Read the model definition and answer for the solid it produces. Units are mm, in the model's axes. Face numbers are marked on the shaded views. A direction names the side the tool comes from. Give positions to 0.01 mm unless a question says otherwise; leave off trailing zeros. Order: outer loops, then holes, each group sorted by start corner. A loop starts at its lowest first (then second) coordinate and runs counter-clockwise, first axis right, second up. Notation, with made-up numbers: (2.25, -37) - (13.25, -37) arc R8 cw to (13.25, -30) - close; hole circle Ø7 at (7, -30). An arc over 180 degrees is marked (long way). Use a Markdown table: item, result. Add a question column.
1. A cutting plane is placed at C-C on x = 36. Determine the outline of the cut face in (y, z), and give its area (3 significant figures).
2. A cutting plane is placed at B-B on z = 13. State how many separate pieces and enclosed holes the cut face has, and give its area (3 significant figures).
3. Consider L1, parallel to X at y = 1.45, z = -4; L2, parallel to Z at x = 62, y = 1.3; L3, parallel to Y at x = 28, z = -6. Determine where each line is inside the solid, lowest interval first.
4. Flat-ended cylindrical pins translate along their axes: P1, Ø9.5, axis at x = 37.36, z = 2.61, coming from the -Y side; P2, Ø1, axis at x = 7.5, z = 11.5, coming from the -Y side. Find the tip coordinate at first contact, or state that the pin passes through.
5. A cutting plane is placed at D-D on x = 67.5. Determine the outline of the cut face in (y, z), and give its area (4 significant figures).
6. Which of the six approach directions +Z, -Z, +X, -X, +Y, -Y give full straight-line access (tool end or side, diameter ignored) to the marked faces 3 and 4?
7. A cutting plane is placed at A-A on x = 17. Determine the outline of the cut face in (y, z).
8. For a pull along Z with two mould halves and no side action, classify the marked faces 1 and 2 as released by +Z, released by -Z, zero draft, split by the parting line, or undercut.
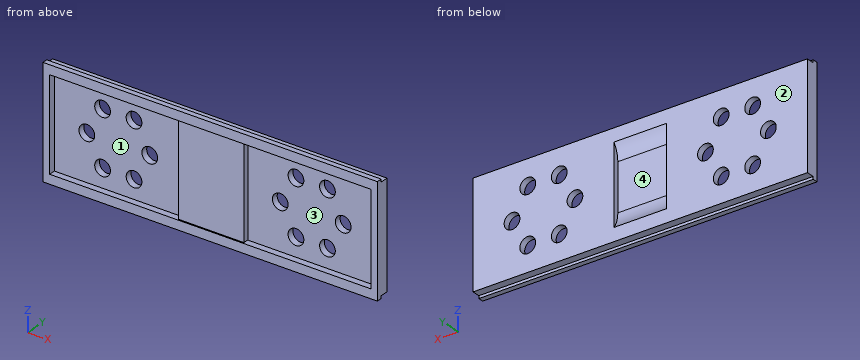
```python
from build123d import *

# Parameters (mm, degrees)
SKETCH1_W           = 127.5
SKETCH1_H           = 42
BOSS_EXTRUDE1_DEPTH = 5
SKETCH2_W           = 127.5
SKETCH2_H           = 1
CUT_EXTRUDE1_DEPTH  = 3
SKETCH7_W           = 20
SKETCH7_H           = 30
CUT_EXTRUDE5_DEPTH  = 2
SHELL8_START        = -14.893859366
SHELL8_DEPTH        = 35
FILLET3_R           = 10
FILLET4_R           = 10
SKETCH10_R          = 3
CUT_EXTRUDE6_DEPTH  = 2.5


# Read off the part's stored shape, not the designer's step: Shell8
with BuildPart() as part:
    # Sketch1 → Boss-Extrude1 (new body)
    with BuildSketch(Plane(origin=(0, 0, 0), x_dir=(1, 0, 0), z_dir=(0, 1, 0))):
        with Locations((12.48267617, -2.606140634)):
            Rectangle(SKETCH1_W, SKETCH1_H)
    extrude(amount=BOSS_EXTRUDE1_DEPTH)

    # Sketch2 → Cut-Extrude1 (cut)
    with BuildSketch(Plane(origin=(0, 5, 0), x_dir=(1, 0, 0), z_dir=(0, 1, 0))):
        with Locations((12.48267617, 17.893859366)):
            Rectangle(SKETCH2_W, SKETCH2_H)
        with Locations((12.48267617, -23.106140634)):
            Rectangle(SKETCH2_W, SKETCH2_H)
    extrude(amount=-CUT_EXTRUDE1_DEPTH, mode=Mode.SUBTRACT)

    # Sketch7 → Cut-Extrude5 (cut)
    with BuildSketch(Plane(origin=(0, 5, 0), x_dir=(1, 0, 0), z_dir=(0, 1, 0))):
        with Locations((12.48267617, -2.606140634)):
            Rectangle(SKETCH7_W, SKETCH7_H)
    extrude(amount=-CUT_EXTRUDE5_DEPTH, mode=Mode.SUBTRACT)

    # Shell8 outline → Shell8 (cut)
    with BuildSketch(Plane.XY.offset(SHELL8_START)):
        Polygon((-0.01732383, 0.5), (-0.01732383, 2.5), (-48.76732383, 2.5), (-48.76732383, 0), (73.73267617, 0), (73.73267617, 2.5), (24.98267617, 2.5), (24.98267617, 0.5), align=None)
    extrude(amount=SHELL8_DEPTH, mode=Mode.SUBTRACT)

    # Fillet3
    # the kernel refuses this fillet: 10 mm, written as the material it adds along each edge
    with BuildSketch(Plane(origin=(37.48267617, 3, 17.606140634), x_dir=(0, 1, 0), z_dir=(-1, 0, 0))) as fillet3_piece_1:
        with BuildLine():
            CenterArc((10, 6), FILLET3_R, 180, 36.869897646)
            Line((0, 6), (-0.2, 6))
            Line((-0.2, 6), (-0.2, 0))
            Line((-0.2, 0), (0, -0.2))
            ThreePointArc((0, -0.2), (1, -0.2), (1.84, -0.12))
            Line((1.84, -0.12), (2, 0))
        make_face()
    extrude(amount=50)

    # Fillet4
    # the kernel refuses this fillet: 10 mm, written as the material it adds along each edge
    with BuildSketch(Plane(origin=(-12.51732383, 3, -12.393859366), x_dir=(0, 0, 1), z_dir=(1, 0, 0))) as fillet4_piece_1:
        with BuildLine():
            CenterArc((6, -10), FILLET4_R, 90, 36.869897646)
            Line((0, -2), (-0.12, -1.84))
            ThreePointArc((-0.12, -1.84), (-0.2, -1), (-0.2, 0))
            Line((-0.2, 0), (0, 0.2))
            Line((0, 0.2), (6, 0.2))
            Line((6, 0.2), (6, 0))
        make_face()
    extrude(amount=50)

    # Sketch10 → Cut-Extrude6 (cut)
    with BuildSketch(Plane(origin=(0, 5, 0), x_dir=(1, 0, 0), z_dir=(0, 1, 0))):
        with Locations(Location((-12.39232383, -2.606140634, 0), (0, 0, 270))):
            Circle(SKETCH10_R)
        with Locations(Location((-18.39232383, -12.998445479, 0), (0, 0, 270))):
            Circle(SKETCH10_R)
        with Locations(Location((-30.39232383, -12.998445479, 0), (0, 0, 270))):
            Circle(SKETCH10_R)
        with Locations(Location((-36.39232383, -2.606140634, 0), (0, 0, 270))):
            Circle(SKETCH10_R)
        with Locations(Location((-30.39232383, 7.786164212, 0), (0, 0, 270))):
            Circle(SKETCH10_R)
        with Locations(Location((-18.39232383, 7.786164212, 0), (0, 0, 270))):
            Circle(SKETCH10_R)
        with Locations(Location((61.35767617, -2.606140634, 0), (0, 0, 270))):
            Circle(SKETCH10_R)
        with Locations(Location((55.35767617, -12.998445479, 0), (0, 0, 270))):
            Circle(SKETCH10_R)
        with Locations(Location((43.35767617, -12.998445479, 0), (0, 0, 270))):
            Circle(SKETCH10_R)
        with Locations(Location((37.35767617, -2.606140634, 0), (0, 0, 270))):
            Circle(SKETCH10_R)
        with Locations(Location((43.35767617, 7.786164212, 0), (0, 0, 270))):
            Circle(SKETCH10_R)
        with Locations(Location((55.35767617, 7.786164212, 0), (0, 0, 270))):
            Circle(SKETCH10_R)
    extrude(amount=-CUT_EXTRUDE6_DEPTH, mode=Mode.SUBTRACT)


solid = part.part
```
Output values:
| question | item | result |
|---|---|---|
| 1 | outline | (0, -18.39) - (2, -18.39) - (2, -17.39) - (5, -17.39) - (5, -0.07) - (2.5, -0.07) - (2.5, -14.89) - (0, -14.89) - close; (0, 20.11) - (2.5, 20.11) - (2.5, 5.28) - (5, 5.28) - (5, 22.61) - (2, 22.61) - (2, 23.61) - (0, 23.61) - close |
| 1 | area | 103 mm² |
| 2 | separate pieces | 5 |
| 2 | enclosed holes | 0 |
| 2 | area | 283 mm² |
| 3 | L1 | -51.27 to -48.77, -0.02 to 24.98, 73.73 to 76.23 |
| 3 | L2 | -18.39 to -14.89, 20.11 to 23.61 |
| 3 | L3 | 2.5 to 5 |
| 4 | P1 | y = 2.5 |
| 4 | P2 | y = 0.5 |
| 5 | outline | (0, -18.39) - (2, -18.39) - (2, -17.39) - (5, -17.39) - (5, 22.61) - (2, 22.61) - (2, 23.61) - (0, 23.61) - (0, 20.11) - (2.5, 20.11) - (2.5, -14.89) - (0, -14.89) - close |
| 5 | area | 116.5 mm² |
| 6 | face 3 | -Y |
| 6 | face 4 | +Y |
| 7 | outline | (0, -18.39) - (2, -18.39) - (2, -17.39) - (5, -17.39) - (5, -12.39) arc R10 cw to (3, -6.39) - (3, 11.61) arc R10 cw to (5, 17.61) - (5, 22.61) - (2, 22.61) - (2, 23.61) - (0, 23.61) - (0, 20.11) - (0.5, 20.11) - (0.5, -14.89) - (0, -14.89) - close |
| 8 | face 1 | undercut |
| 8 | face 2 | zero draft |
